```python
from build123d import *

# Parameters (mm, degrees)
PAD_DEPTH       = 30
SKETCH001_R     = 2
POCKET_DEPTH    = 50
SKETCH002_W     = 81.7157287525
SKETCH002_H     = 17.25
SKETCH002_W_2   = 73.7157287525
SKETCH002_H_2   = 5.5
POCKET001_DEPTH = 50
SKETCH003_W     = 6
SKETCH003_H     = 73.7157287525
POCKET002_DEPTH = 50
FILLET_R        = 3


with BuildPart() as part:
    # Sketch → Pad (new body, symmetric)
    with BuildSketch(Plane.YZ):
        Polygon((64.5161954169, 20), (64.5161954169, 0), (20, 0), (0, 70), (0, 160), (20, 160), (20, 70.8066839593), (34.5161954169, 20), align=None)
    extrude(amount=PAD_DEPTH, both=True)

    # Sketch001 (on Face3 of Pad) → Pocket (cut)
    with BuildSketch(Plane(origin=(0, 0, 20), x_dir=(0, -1, 0), z_dir=(0, 0, 1))):
        with Locations((-56.5161954169, -15)):
            Circle(SKETCH001_R)
        with Locations((-56.5161954169, 15)):
            Circle(SKETCH001_R)
        with Locations((-41.5161954169, 15)):
            Circle(SKETCH001_R)
        with Locations((-41.5161954169, -15)):
            Circle(SKETCH001_R)
    extrude(amount=-POCKET_DEPTH, mode=Mode.SUBTRACT)

    # Sketch002 (on Face6 of Pocket) → Pocket001 (cut)
    with BuildSketch(Plane(origin=(0, 0, 0), x_dir=(0, 0, -1), z_dir=(0, -1, 0))):
        with Locations((-119.1421356237, 21.375)):
            Rectangle(SKETCH002_W, SKETCH002_H)
        with Locations((-119.1421356237, -21.375)):
            Rectangle(SKETCH002_W, SKETCH002_H)
        with Locations((-115.1421356237, 0)):
            Rectangle(SKETCH002_W_2, SKETCH002_H_2)
    extrude(amount=-POCKET001_DEPTH, mode=Mode.SUBTRACT)

    # Sketch003 (on Face8 of Pocket001) → Pocket002 (cut)
    with BuildSketch(Plane.YZ.offset(12.75)):
        with Locations((9, 115.1421356237)):
            Rectangle(SKETCH003_W, SKETCH003_H)
    extrude(amount=-POCKET002_DEPTH, mode=Mode.SUBTRACT)

    # Fillet
    fillet_edges = [part.edges().sort_by_distance(p)[0] for p in [
        (30, 27.258098, 45.403342),
        (-30, 27.258098, 45.403342),
        (30, 49.516195, 20),
        (0, 64.516195, 20),
        (-30, 64.516195, 10),
        (-30, 49.516195, 20),
        (30, 64.516195, 10),
        (12.75, 20, 119.142136),
        (-12.75, 20, 119.142136),
        (0, 20, 160),
        (12.75, 10, 160),
        (0, 0, 160),
        (-12.75, 10, 160),
        (12.75, 0, 119.142136),
        (30, 10, 78.284271),
        (21.375, 0, 78.284271),
        (-12.75, 0, 119.142136),
        (-30, 10, 78.284271),
        (-21.375, 0, 78.284271),
        (-30, 0, 74.142136),
        (-30, 10, 35),
        (0, 0, 70),
        (30, 10, 35),
        (30, 0, 74.142136),
    ]]
    fillet(fillet_edges, radius=FILLET_R)


solid = part.part
```
For this review, take the finished solid that the model builds, in its own axes (mm). A direction names the side the tool comes from. Round coordinates to 2 decimals unless told otherwise and drop trailing zeros. Write each loop counter-clockwise with the first axis right and the second up, starting at its lowest first coordinate (ties: lowest second). Pieces come first, ordered by that corner, then holes. Notation, with made-up numbers: (50, 63) -> (99, 63) arc R19 cw to (99, 69) -> close; hole circle Ø3 at (23, 10.25). An arc over 180 degrees is marked (long way). One line per question, with ' | ' between items. Start each with the question number.
1) Add section D-D (x = -22). Write out the cut boundary in (y, z).
2) Add section C-C (x = -8). Write out the cut boundary in (y, z), and give its area (3 significant figures).
3) Wall thickness on line 1 along Y through (x, z) = (-8.5, 85); line 2 along X through (y, z) = (13, 98); line 3 along Z through (x, y) = (2, 38.5): over which ranges is each line inside the solid? List them lowest first.
4) Mouldability with a two-part tool opening along Y and no side actions: class faces 1 (the flat face through (0, 10, 78.284)), 2 (the flat face through (2.75, 3, 116)), 3 (the cylindrical face through (-11.89, 19.1, 117.09)), 4 (the flat face through (4, 0, 104)) as +Y half, -Y half, draft (parallel to the pull), parting line (faces both ways), or undercut.
5) For pin 1 Ø11 at (x, z) = (10, 132) entering from +Y; pin 2 Ø9 at (y, z) = (15.5, 128.5) entering from -X; pin 3 Ø10 at (x, z) = (-4, 41.5) entering from -Y, all flat-tipped, find the tip position at first contact; note any pin that passes through.
6) Add section A-A (x = -15). Write out the cut boundary in (y, z), and give its area (3 significant figures).
7) Add section B-B (z = 98). Write out the cut boundary in (x, y), and give its area (3 significant figures).
8) Machinability: for faces 5 (the cylindrical face through (-18.254, 0.855, 77.382)), 6 (the flat face through (0, 10, 152)), 7 (the cylindrical face through (11.85, 0.86, 115.57)), 8 (the flat face through (12.75, 13, 118)), which of the approach directions +Z, -Z, +X, -X, +Y, -Y give a long, thin tool a straight path to every point of the face, cutting with its end or side? Answer none if there is none.
Reported:
1) outline: (0, 70.42) arc R3 ccw to (0.12, 69.6) -> (20, 0) -> (64.52, 0) -> (64.52, 17) arc R3 ccw to (61.52, 20) -> (34.52, 20) -> (20, 70.81) -> (20, 78.28) -> (3, 78.28) arc R3 ccw to (0, 75.28) -> close
2) outline: (0, 70.42) arc R3 ccw to (0.12, 69.6) -> (20, 0) -> (64.52, 0) -> (64.52, 17) arc R3 ccw to (61.52, 20) -> (34.52, 20) -> (20, 70.81) -> (20, 157) arc R3 ccw to (17, 160) -> (3, 160) arc R3 ccw to (0, 157) -> close; hole (6, 78.28) -> (12, 78.28) -> (12, 152) -> (6, 152) -> close | area: 3,310 mm²
3) line 1: y = 0 to 6, 12 to 20 | line 2: x = -12.75 to -2.75, 2.75 to 12.75 | line 3: z = 0 to 20
4) face 1: undercut | face 2: draft | face 3: +Y half | face 4: -Y half
5) pin 1: stops at y = 20 | pin 2: stops at x = -12.75 | pin 3: stops at y = 6.71
6) outline: (0, 70.42) arc R3 ccw to (0.12, 69.6) -> (20, 0) -> (39.52, 0) -> (39.52, 20) -> (34.52, 20) -> (20, 70.81) -> (20, 78.28) -> (3, 78.28) arc R3 ccw to (0, 75.28) -> close; (43.52, 0) -> (54.52, 0) -> (54.52, 20) -> (43.52, 20) -> close; (58.52, 0) -> (64.52, 0) -> (64.52, 17) arc R3 ccw to (61.52, 20) -> (58.52, 20) -> close | area: 1,960 mm²
7) outline: (-12.75, 3) arc R3 ccw to (-9.75, 0) -> (-2.75, 0) -> (-2.75, 6) -> (-12.75, 6) -> close; (-12.75, 12) -> (-2.75, 12) -> (-2.75, 20) -> (-9.75, 20) arc R3 ccw to (-12.75, 17) -> close; (2.75, 0) -> (9.75, 0) arc R3 ccw to (12.75, 3) -> (12.75, 6) -> (2.75, 6) -> close; (2.75, 12) -> (12.75, 12) -> (12.75, 17) arc R3 ccw to (9.75, 20) -> (2.75, 20) -> close | area: 272 mm²
8) face 5: +Z, -X, -Y | face 6: none | face 7: +Z, +X, -Y | face 8: +Z, +X, +Y, -Y
